The model under review builds one solid part; all positions refer to its coordinate system, in mm. A direction names the side the tool comes from. Round coordinates to 2 decimals unless told otherwise and drop trailing zeros. Write each loop counter-clockwise with the first axis right and the second up, starting at its lowest first coordinate (ties: lowest second). Pieces come first, ordered by that corner, then holes.
Item 1: Add section B-B (y = 4.5). Give the boundary of the cut face in (x, z).
Item 2: Add section C-C (z = -5). Give the boundary of the cut face in (x, y).
Item 3: Add section D-D (y = 9.5). Give the boundary of the cut face in (x, z).
Item 4: Add section A-A (x = 4). Give the boundary of the cut face in (y, z).
Item 5: To check wall thickness, follow L1, parallel to X at y = 6, z = -17; L2, parallel to Y at x = 13, z = -4; L3, parallel to Z at x = 12.3, y = 4.7. State the ranges of each line that lie inside material, in increasing order.
Item 6: Machinability: for faces 1 (the face through (8, 7, -11)), 2 (the face through (8, 5, -7)), 3 (the face through (11.65, 5.27, -14.07)), which of the approach directions +Z, -Z, +X, -X, +Y, -Y give a long, thin tool a straight path to every point of the face, cutting with its end or side? Answer none if there is none.
Item 7: Draft analysis for pull direction Y (two halves, no side actions). For faces 4 (the face through (14.4, 19, -3)), 5 (the face through (8, 0, -10)), 6 (the face through (15, 14, 0)), state which applies: +Y half, -Y half, draft (parallel to the pull), parting line (faces both ways), or undercut.
Item 8: Clearance check with flat-ended pins moving along their axes: pin 1 Ø1.2 at (x, z) = (4, -17) entering from +Y; pin 2 Ø8 at (x, z) = (12.3, -17) entering from +Y; pin 3 Ø3.5 at (x, z) = (4, -17) entering from +Y; pin 4 Ø0.6 at (x, y) = (8, 5) entering from +Z. State where each tip first meets the part, or that it passes through.
Autodesk Inventor part; units mm, degrees
ref_plane "YZ Plane" through (0, 0, 0) normal (1, 0, 0) x (0, 1, 0)
ref_plane "XZ Plane" through (0, 0, 0) normal (0, 1, 0) x (-1, 0, 0)
ref_plane "XY Plane" through (0, 0, 0) normal (0, 0, 1) x (1, 0, 0)
sketch "Sketch1" plane through (0, 0, 0) normal (1, 0, 0) x (0, 1, 0)
  line L0 (34.6, 0) -> (0, 0)
  line L1 (0, 0) -> (0, -40)
  line L2 (7, -40) -> (7, -5)
  line L3 (7, -5) -> (34.6, -5)
  line L4 (34.6, -5) -> (34.6, 0)
  line L5 (7, -40) -> (0, -40)
  dimension "d0" = 0
  dimension "d1" = 0
  dimension "d2" = 5
  dimension "d3" = 7
  dimension "d5" = 40
  dimension "d6" = 34.6
extrude "Extrusion1" add sketch "Sketch1" along normal blind 16.3
sketch "Sketch2" plane through (0, 7, -5) normal (0, 1, 0) x (1, 0, 0)
  line L0 (16.3, 35) -> (16.3, 0)
  line L1 (0, -5) -> (16.3, -5)
  circle A0 centre (12.3, 12) radius 1
  line L2 (12.3, 5) -> (12.3, 12) construction
  circle A1 centre (4, 12) radius 1
  line L3 (0, 35) -> (0, 0)
  line L4 (0, 0) -> (16.3, 0)
  dimension "d9" = 4
  dimension "d31" = 2
  dimension "d46" = 4
  dimension "d47" = 12
  dimension "d48" = 0
extrude "Extrusion2" cut sketch "Sketch2" against normal through all
sketch "Sketch3" plane through (0, 7, -5) normal (0, 0, -1) x (-1, 0, 0)
  line L0 (0, 0) -> (-16.3, 0)
  line L1 (-14.4, 0) -> (-1.9, 0)
  line L2 (-1.9, 0) -> (-1.9, 23)
  line L3 (-1.9, 23) -> (-14.4, 23)
  line L4 (-14.4, 23) -> (-14.4, 0)
  line L5 (0, 0) -> (0, 27.6)
  point P0 (0, -7)
  dimension "d14" = 23
  dimension "d15" = 12.5
  dimension "d16" = 1.9
extrude "Extrusion3" cut sketch "Sketch3" against normal blind 16.3
sketch "Sketch5" plane through (0, 7, -5) normal (0, 0, -1) x (-1, 0, 0)
  line L0 (0, 27.6) -> (-16.3, 27.6)
  line L1 (-16.3, 27.6) -> (0, 27.6)
  line L2 (0, 27.6) -> (0, 0)
  line L3 (0, 0) -> (-1.9, 0)
  line L4 (-14.4, 23) -> (-14.4, 0)
  line L5 (-14.4, 23) -> (-14.4, 0)
  line L6 (-14.4, 0) -> (-16.3, 0)
  line L7 (-16.3, 0) -> (-16.3, 27.6)
  line L8 (-14.4, 23) -> (-1.9, 23)
  line L9 (-1.9, 23) -> (-1.9, 0)
  line L10 (-1.9, 23) -> (-1.9, 0)
  line L11 (-14.4, 23) -> (-1.9, 23)
  point P0 (0, -7)
  dimension "d26" = 0
  dimension "d27" = 0
  dimension "d28" = 1.9
extrude "Extrusion5" add sketch "Sketch5" along normal blind 4
sketch "Sketch4" plane through (0, 0, 0) normal (0, 0, 1) x (1, 0, 0)
  circle A0 centre (8.15, 32.5) radius 1
  circle A1 centre (8.15, 4.5) radius 1
  line L0 (1.9, 30) -> (14.4, 30)
  line L1 (14.4, 7) -> (1.9, 7)
  line L2 (0, 34.6) -> (0, 0)
  line L3 (16.3, 34.6) -> (16.3, 0)
  dimension "d19" = 2.5
  dimension "d20" = 2.5
  dimension "d21" = 2
  dimension "d22" = 8.15
  dimension "d23" = 8.15
extrude "Extrusion4" cut sketch "Sketch4" against normal blind 7
sketch "Sketch7" plane through (0, 34.6, 0) normal (0, 1, 0) x (1, 0, 0)
  line L0 (16.3, 0) -> (16.3, 9)
  line L1 (0, 0) -> (0, 9)
  line L2 (16.3, 9) -> (0, 9)
  line L3 (0, 9) -> (0, 6)
  line L4 (0, 6) -> (16.3, 6)
  line L5 (16.3, 6) -> (16.3, 9)
  line L6 (0, 0) -> (16.3, 0)
  dimension "d40" = 6
extrude "Extrusion7" cut sketch "Sketch7" against normal up to surface (27.6 mm away) contours L4 L1 L2 L0
sketch "Sketch8" plane through (0, 7, -40) normal (0, 1, 0) x (1, 0, 0)
  line L0 (0, 0) -> (16.3, 0)
  line L1 (0, 0) -> (0, -34)
  line L2 (16.3, 0) -> (0, 0)
  line L3 (0, 0) -> (0, -19)
  line L4 (0, -19) -> (16.3, -19)
  line L5 (16.3, -19) -> (16.3, 0)
  circle A0 centre (12.3, -23) radius 1
  point P0 (0, -40)
  dimension "d43" = 4
extrude "Extrusion8" cut sketch "Sketch8" against normal blind 10 contours L0 L5 L4 L1
sketch "Sketch9" plane through (1.9, 7, 0) normal (0, 1, 0) x (1, 0, 0)
  circle A0 centre (2.1, 17) radius 1
  circle A1 centre (10.4, 17) radius 1
  circle A2 centre (2.1, 17) radius 3
  circle A3 centre (10.4, 17) radius 3
  point P0 (-1.9, 0)
  dimension "d49" = 6
  dimension "d50" = 6
extrude "Extrusion9" cut sketch "Sketch9" against normal blind 3.5
equation "\"d50\" = d49"
properties part number "ServoHolder_3DPrint"
Numbers:
1. outline: (0, -21) - (16.3, -21) - (16.3, 0) - (9.15, 0) - (9.15, -7) - (7.15, -7) - (7.15, 0) - (0, 0) - close; hole circle Ø6 at (4, -17); hole circle Ø6 at (12.3, -17)
2. outline: (0, 0) - (16.3, 0) - (16.3, 34.6) - (0, 34.6) - close; hole (1.9, 7) - (14.4, 7) - (14.4, 30) - (1.9, 30) - close; hole circle Ø2 at (8.15, 4.5); hole circle Ø2 at (8.15, 32.5)
3. outline: (0, -6) - (1.9, -6) - (1.9, 0) - (0, 0) - close; (14.4, -6) - (16.3, -6) - (16.3, 0) - (14.4, 0) - close
4. outline: (0, -21) - (7, -21) - (7, -20) - (3.5, -20) - (3.5, -18) - (0, -18) - close; (0, -16) - (3.5, -16) - (3.5, -14) - (7, -14) - (7, 0) - (0, 0) - close; (30, -6) - (34.6, -6) - (34.6, 0) - (30, 0) - close
5. L1: x = 0 to 1, 7 to 9.3, 15.3 to 16.3
5. L2: y = 0 to 7, 30 to 34.6
5. L3: z = -21 to -20, -14 to 0
6. face 1: -Z
6. face 2: +Z
6. face 3: +Y
7. face 4: undercut
7. face 5: -Y half
7. face 6: draft
8. pin 1: passes through
8. pin 2: stops at y = 7
8. pin 3: stops at y = 3.5
8. pin 4: stops at z = -7
